Read the model definition and answer for the solid it produces. Units are mm, in the model's axes. Face numbers are marked on the shaded views. A direction names the side the tool comes from. Give positions to 0.01 mm unless a question says otherwise; leave off trailing zeros. Order: outer loops, then holes, each group sorted by start corner. A loop starts at its lowest first (then second) coordinate and runs counter-clockwise, first axis right, second up.
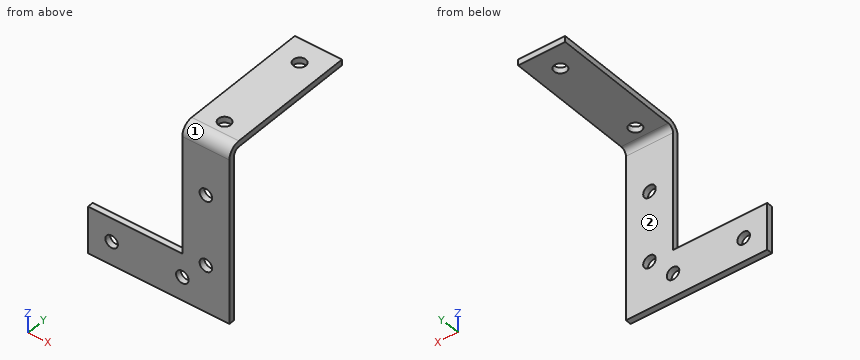
Autodesk Inventor part; units mm, degrees
ref_plane "YZ Plane" through (0, 0, 0) normal (1, 0, 0) x (0, 1, 0)
ref_plane "XZ Plane" through (0, 0, 0) normal (0, 1, 0) x (-1, 0, 0)
ref_plane "XY Plane" through (0, 0, 0) normal (0, 0, 1) x (1, 0, 0)
sketch "Sketch1" plane through (0, 0, 0) normal (0, 1, 0) x (-1, 0, 0)
  line L0 (0, 0) -> (0, 76.2)
  line L1 (25.4, 76.2) -> (25.4, 25.4)
  line L2 (25.4, 25.4) -> (76.2, 25.4)
  line L3 (76.2, 25.4) -> (76.2, 0)
  line L4 (76.2, 0) -> (0, 0)
  line L5 (25.4, 25.4) -> (0, 0) construction
  circle A0 centre (12.7, 63.5) radius 3.3782
  circle A1 centre (12.7, 25.4) radius 3.3782
  circle A2 centre (25.4, 12.7) radius 3.3782
  circle A3 centre (63.5, 12.7) radius 3.3782
  line L6 (25.4, 76.2) -> (25.4, 95.25)
  line L7 (25.4, 95.25) -> (0, 95.25)
  line L8 (0, 95.25) -> (0, 76.2)
  point P0 (0, 0)
  dimension "d0" = 76.2
  dimension "d1" = 25.4
  dimension "d2" = 50.8
  dimension "d3" = 50.8
  dimension "d4" = 25.4
  dimension "d5" = 6.7564
  dimension "d6" = 6.7564
  dimension "d7" = 6.7564
  dimension "d8" = 6.7564
  dimension "d9" = 12.7
  dimension "d10" = 0
  dimension "d11" = 12.7
  dimension "d12" = 12.7
  dimension "d13" = 12.7
  dimension "d15" = 12.7
  dimension "d17" = 19.05
extrude "Plate1" add sketch "Sketch1" along normal blind 3.175
sketch "Sketch2" plane through (0, 0, 92.075) normal (0, 0, 1) x (1, 0, 0)
  line L0 (-25.4, 0) -> (0, 0)
  line L1 (0, 0) -> (0, 76.2)
  line L2 (0, 76.2) -> (-25.4, 76.2)
  line L3 (-25.4, 76.2) -> (-25.4, 0)
edge flange "Flange1" height 76.2 angle 90 thickness 3.175 bend radius 3.175 thickness toward (0, 0, 1) relief tear relief width 3.175 relief depth 1.5875 edges at (-12.7, 3.175, 95.25) wall of the first edge with corners at (-25.4, 0, 92.075) (0, 0, 92.075) (0, 76.2, 92.075) (-25.4, 76.2, 92.075)
bend "Bend1"
corner "Corner1"
sketch "Sketch3" plane through (0, 76.2, 92.075) normal (0, 0, -1) x (-1, 0, 0)
  line L0 (25.4, 0) -> (0, 0)
  circle A0 centre (12.7, -12.7) radius 3.3782
  circle A1 centre (12.7, -63.5) radius 3.3782
  point P0 (0, -76.2)
  dimension "d29" = 6.7564
  dimension "d30" = 6.7564
  dimension "d31" = 12.7
  dimension "d32" = 50.8
extrude "Cut1" cut sketch "Sketch3" against normal blind 3.175
equation "\"d33\" = Thickness"
equation "\"d19\" = BendReliefWidth"
equation "\"d20\" = BendReliefDepth"
equation "\"d21\" = MinimumRemnant"
equation "\"d22\" = BendRadius"
equation "\"d25\" = BendRadius"
equation "\"d26\" = CornerReliefSize"
equation "\"d27\" = GapSize"
equation "\"d28\" = JacobiRadiusSize"
equation "\"BendRadius\" = Thickness"
equation "\"BendReliefWidth\" = Thickness"
equation "\"BendReliefDepth\" = 0.5 * Thickness"
equation "\"CornerReliefSize\" = 4 * Thickness"
equation "\"MinimumRemnant\" = 2 * Thickness"
equation "\"TransitionRadius\" = BendRadius"
equation "\"JacobiRadiusSize\" = BendRadius"
equation "\"GapSize\" = Thickness"
equation "\"d18\" = BendRadius"
properties part number "Gusset 2"
1) Given pin 1 (11 mm diameter, centred on x = -12.7, y = 63.5, fed in from -Z) (3 decimals); pin 2 (3.5 mm diameter, centred on x = -50.5, y = 1, fed in from +Z); pin 3 (8 mm diameter, centred on x = -63.5, z = 12.7, fed in from +Y) (3 decimals), each flat-ended and moving along its own axis, determine where each tip first touches the part or whether it passes through.
Final values:
pin 1: stops at z = 92.075
pin 2: stops at z = 25.4
pin 3: stops at y = 3.175
2) The part is cut by section A-A on x = -12.7. Determine the outline of the cut face in (y, z) (3 decimals), and give its area (3 significant figures).
Final values:
outline: (0, 0) - (3.175, 0) - (3.175, 22.022) - (0, 22.022) - close; (0, 28.778) - (3.175, 28.778) - (3.175, 60.122) - (0, 60.122) - close; (0, 66.878) - (3.175, 66.878) - (3.175, 88.9) arc R3.175 cw to (6.35, 92.075) - (9.322, 92.075) - (9.322, 95.25) - (6.35, 95.25) arc R6.35 ccw to (0, 88.9) - close; (16.078, 92.075) - (60.122, 92.075) - (60.122, 95.25) - (16.078, 95.25) - close; (66.878, 92.075) - (76.2, 92.075) - (76.2, 95.25) - (66.878, 95.25) - close
area: 442 mm2
3) The part is cut by section C-C on z = 63.5. Determine the outline of the cut face in (x, y) (3 decimals).
Final values:
outline: (-25.4, 0) - (-16.078, 0) - (-16.078, 3.175) - (-25.4, 3.175) - close; (-9.322, 0) - (0, 0) - (0, 3.175) - (-9.322, 3.175) - close
4) A tool of negligible diameter and unlimited length cuts with its end or side. For the marked faces 1 and 2, from which of +Z, -Z, +X, -X, +Y, -Y can it reach the whole face along a straight path? Write none if from no direction.
Final values:
face 1: +Z, +X, -X, -Y
face 2: -Z, +X, -X, +Y
5) The part is cut by section B-B on y = 63.5. Determine the outline of the cut face in (x, z) (3 decimals), and give its area (3 significant figures).
Final values:
outline: (-25.4, 92.075) - (-16.078, 92.075) - (-16.078, 95.25) - (-25.4, 95.25) - close; (-9.322, 92.075) - (0, 92.075) - (0, 95.25) - (-9.322, 95.25) - close
area: 59.2 mm2
6) The part is cut by section D-D on y = 20.5. Determine the outline of the cut face in (x, z) (3 decimals).
Final values:
outline: (-25.4, 92.075) - (0, 92.075) - (0, 95.25) - (-25.4, 95.25) - close
7) Consider L1, parallel to Y at x = -12.7, z = 94; L2, parallel to Y at x = -12.7, z = 93.55; L3, parallel to Z at x = -63.5, y = 1.2. Determine where each line is inside the solid, lowest interval first.
Final values:
L1: y = 2.57 to 9.32, 16.08 to 60.12, 66.88 to 76.2
L2: y = 2.03 to 9.32, 16.08 to 60.12, 66.88 to 76.2
L3: z = 0 to 9.32, 16.08 to 25.4
